Autodesk Inventor part; units mm, degrees
ref_plane "YZ Plane" through (0, 0, 0) normal (1, 0, 0) x (0, 1, 0)
ref_plane "XZ Plane" through (0, 0, 0) normal (0, 1, 0) x (-1, 0, 0)
ref_plane "XY Plane" through (0, 0, 0) normal (0, 0, 1) x (1, 0, 0)
sketch "Esboço1" plane through (0, 0, 0) normal (0, 0, 1) x (1, 0, 0)
  circle A0 centre (0, 0) radius 3
  circle A1 centre (0, 0) radius 8
  dimension "d0" = 6
  dimension "d1" = 16
extrude "Extrusão1" add sketch "Esboço1" along normal mid plane 8
chamfer "Chanfro1" distance 0.3 angle 45 4 edges at (-3, 0, 4) (-8, 0, 4) (-8, 0, -4) (-3, 0, -4)
Build history of the part. All positions in model axes, mm. Give positions to 0.01 mm unless a question says otherwise; leave off trailing zeros. Loops run counter-clockwise (first coordinate to the right, second up) from the corner with the lowest first, then second, coordinate; pieces in that order, holes last. Notation, with made-up numbers: (84.25, -17.5) - (104.25, -17.5) arc R28 cw to (104.25, 13.5) - close; hole circle Ø5 at (78, 2). An arc over 180 degrees is marked (long way). Write item = value, one per line. Start each with the question number.
1) Probe probe 1 along Y at (x, z) = (0, 1); probe 2 along Y at (x, z) = (1.75, -2.5). List the from-to ranges inside material, lowest first. Write a range as from..to.
2) Band-saw the part on C-C on z = -3. Give the cut face in (x, y).
3) Drop flat-ended pins along their axis: pin 1 Ø4 at (y, z) = (2.5, 1) entering from +X; pin 2 Ø1 at (x, z) = (6, -2.5) entering from +Y; pin 3 Ø1 at (x, z) = (5.5, 1) entering from +Y (3 decimals). Give the stop position or say it passes through.
4) Pull direction Y, two halves, no side cores. Call faces 1 (the cylindrical face through (-3, 0, 0)), 2 (the cylindrical face through (-1.73, -7.81, 0.05)), 3 (the flat face through (3, -2, -4)): +Y half, -Y half, draft (parallel to the pull), parting line (faces both ways), or undercut.
5) Band-saw the part on A-A on y = 0. Give the cut face in (x, z), plus the area to 3 significant figures.
Final values:
q1.probe_1 = -8..-3, 3..8
q1.probe_2 = -7.81..-2.44, 2.44..7.81
q2.outline = circle Ø16 at (0, 0); hole circle Ø6 at (0, 0)
q3.pin_1 = 7.98
q3.pin_2 = 5.81
q3.pin_3 = 6.245
q4.face_1 = undercut
q4.face_2 = parting line
q4.face_3 = draft
q5.outline = (-8, -3.7) - (-7.7, -4) - (-3.3, -4) - (-3, -3.7) - (-3, 3.7) - (-3.3, 4) - (-7.7, 4) - (-8, 3.7) - close; (3, -3.7) - (3.3, -4) - (7.7, -4) - (8, -3.7) - (8, 3.7) - (7.7, 4) - (3.3, 4) - (3, 3.7) - close
q5.area = 79.6 mm²
